Read the model definition and answer for the solid it produces. Units are mm, in the model's axes. A direction names the side the tool comes from. Coordinates: 2 decimals unless noted, no trailing zeros. Write each loop counter-clockwise with the first axis right and the second up, starting at its lowest first coordinate (ties: lowest second). Pieces come first, ordered by that corner, then holes. Notation, with made-up numbers: (-29.75, 55.5) -> (-10.75, 55.5) arc R6 cw to (-10.75, 64.5) -> close; hole circle Ø5 at (-7, -30.5). An arc over 180 degrees is marked (long way). Answer in a Markdown table with one row per item. Add a question column.
Item 1: Straight lines are drawn through the part: line 1 (Y direction, x = 0, z = 182); line 2 (Y direction, x = 12, z = 181.5); line 3 (Y direction, x = 15.75, z = 182.5). For each, find the intervals that lie inside material, in ascending order. Write a range as from..to.
Item 2: Given pin 1 Ø1.5 at (y, z) = (10, 204.5) entering from -X; pin 2 Ø8.5 at (y, z) = (-12.5, 183.5) entering from +X; pin 3 Ø0.5 at (x, z) = (19, 199) entering from -Y; pin 4 Ø2.5 at (x, y) = (-16.5, -11) entering from -Z, each flat-ended and moving along its own axis, determine where each tip first touches the part or whether it passes through.
Item 3: Section A-A on x = 0 is taken. Count the separate pieces of the cut face and the enclosed holes in it, then the cut area to 3 significant figures.
Item 4: Which of the six approach directions +Z, -Z, +X, -X, +Y, -Y give full straight-line access (tool end or side, diameter ignored) to faces 1 (the face through (16, -12, 187.3)), 2 (the face through (22, -7, 182.3)), 3 (the face through (19.069, -3.542, 188.468))?
Item 5: For a pull along Y with two mould halves and no side action, classify faces 4 (the face through (23, 3.7, 196)), 5 (the face through (-23.877, -1.051, 186.742)), 6 (the face through (17, -2, 188)) as +Y half, -Y half, draft (parallel to the pull), parting line (faces both ways), or undercut.
Item 6: Section D-D on z = 201 is taken. Write down the section's boundary in (x, y).
Item 7: Section C-C on z = 205.3 is taken. Write down the section's boundary in (x, y), then the cut area to 3 significant figures.
```python
from build123d import *

# Parameters (mm, degrees)
PAD022_DEPTH    = 10
CHAMFER009_SIZE = 0.5
SKETCH040_R     = 23.9
SKETCH040_R_2   = 22.6
PAD023_DEPTH    = 24
SKETCH041_R     = 23.5
SKETCH041_W     = 20
SKETCH041_H     = 7.75
PAD024_DEPTH    = 24
SKETCH042_R     = 23.9
PAD025_DEPTH    = 4
CHAMFER010_SIZE = 0.5
SKETCH043_R     = 1.5
POCKET013_DEPTH = 15
SKETCH044_R     = 1
POCKET014_DEPTH = 100
SKETCH045_R     = 1.25
POCKET015_DEPTH = 15
SKETCH052_W     = 5
SKETCH052_H     = 18
POCKET019_DEPTH = 41
SKETCH055_W     = 10
SKETCH055_H     = 14
POCKET021_DEPTH = 33


with BuildPart() as part:
    # Sketch039 → Pad022 (new body)
    with BuildSketch(Plane.XY):
        with BuildLine():
            ThreePointArc((-14.5, 18.872997), (-23.8, 0), (-14.5, -18.872997))
            Line((-14.5, -18.872997), (14.5, -18.872997))
            ThreePointArc((14.5, -18.872997), (23.8, 0), (14.5, 18.872997))
            Line((-14.5, 18.872997), (14.5, 18.872997))
        make_face()
        with BuildLine():
            ThreePointArc((-13.831702, 17.872997), (-22.6, 0), (-13.831702, -17.872997))
            Line((13.831702, -17.872997), (-13.831702, -17.872997))
            ThreePointArc((13.831702, -17.872997), (22.6, 0), (13.831702, 17.872997))
            Line((-13.831702, 17.872997), (13.831702, 17.872997))
        make_face(mode=Mode.SUBTRACT)
    extrude(amount=PAD022_DEPTH)

    # Chamfer009
    chamfer009_edges = [part.edges().sort_by_distance(p)[0] for p in [
        (0, -18.872997, 10),
        (0, 18.872997, 10),
    ]]
    chamfer(chamfer009_edges, length=CHAMFER009_SIZE)

    # Sketch040 (on Face4 of Chamfer009) → Pad023 (join)
    with BuildSketch(Plane(origin=(0, 0, 0), x_dir=(1, 0, 0), z_dir=(0, 0, -1))):
        Circle(SKETCH040_R)
        Circle(SKETCH040_R_2, mode=Mode.SUBTRACT)
    extrude(amount=PAD023_DEPTH)

    # Sketch041 (on Face4 of Pad023) → Pad024 (join)
    with BuildSketch(Plane.XY):
        Circle(SKETCH041_R)
        with BuildLine():
            Line((-22.528563, 1.795511), (-18, 0.997003))
            Line((-18, 0.997003), (-18, -0.002997))
            Line((-18, -0.002997), (-20, -0.002997))
            Line((-20, -0.002997), (-20, -2.002997))
            Line((-18, -2.002997), (-20, -2.002997))
            Line((-18, -2.002997), (-18, -3.002997))
            Line((-18, -3.002997), (-22.225594, -4.096705))
            ThreePointArc((-22.225594, -4.096705), (-21.597921, -6.655058), (-20.676821, -9.122997))
            Line((-20.676821, -9.122997), (20.676821, -9.122997))
            ThreePointArc((20.676821, -9.122997), (21.597428, -6.656659), (22.224986, -4.1))
            Line((16, -3), (22.224986, -4.1))
            Line((16, -2), (16, -3))
            Line((18, -2), (16, -2))
            Line((18, 0), (18, -2))
            Line((18, 0), (16, 0))
            Line((16, 0), (16, 1))
            Line((16, 1), (22.528205, 1.8))
            ThreePointArc((22.528205, 1.8), (19.877022, 10.754719), (13.831702, 17.872997))
            Line((13.831702, 17.872997), (-13.831702, 17.872997))
            ThreePointArc((-13.831702, 17.872997), (-19.878094, 10.752739), (-22.528563, 1.795511))
        make_face(mode=Mode.SUBTRACT)
        with Locations((0, -13.997997)):
            Rectangle(SKETCH041_W, SKETCH041_H, mode=Mode.SUBTRACT)
    extrude(amount=-PAD024_DEPTH)

    # Sketch042 (on Face49 of Pad024) → Pad025 (join)
    with BuildSketch(Plane(origin=(0, 0, -24), x_dir=(1, 0, 0), z_dir=(0, 0, -1))):
        Circle(SKETCH042_R)
    extrude(amount=PAD025_DEPTH)

    # Chamfer010
    chamfer010_edges = [part.edges().sort_by_distance(p)[0] for p in [
        (-23.9, 0, -28),
    ]]
    chamfer(chamfer010_edges, length=CHAMFER010_SIZE)

    # Sketch043 (on Face4 of Chamfer010) → Pocket013 (cut)
    with BuildSketch(Plane(origin=(0, 0, -28), x_dir=(1, 0, 0), z_dir=(0, 0, -1))):
        with Locations((-15.75, 11.916375)):
            Circle(SKETCH043_R)
        with Locations((15.75, 11.916375)):
            Circle(SKETCH043_R)
        with Locations((0, -19.75)):
            Circle(SKETCH043_R)
    extrude(amount=-POCKET013_DEPTH, mode=Mode.SUBTRACT)

    # Sketch044 (on Face9 of Pocket013) → Pocket014 (cut)
    with BuildSketch(Plane.XZ.offset(18.872997)):
        with Locations((0, 5)):
            Circle(SKETCH044_R)
    extrude(amount=-POCKET014_DEPTH, mode=Mode.SUBTRACT)

    # Sketch045 (on Face29 of Pocket014) → Pocket015 (cut)
    with BuildSketch(Plane.XY):
        with Locations((12.5, -15)):
            Circle(SKETCH045_R)
        with Locations((-12.5, -15)):
            Circle(SKETCH045_R)
    extrude(amount=-POCKET015_DEPTH, mode=Mode.SUBTRACT)

    # Sketch052 → Pocket019 (cut)
    with BuildSketch(Plane.YZ):
        with Locations((-6.6, -9)):
            Rectangle(SKETCH052_W, SKETCH052_H)
    extrude(amount=POCKET019_DEPTH, mode=Mode.SUBTRACT)

    # Sketch055 → Pocket021 (cut)
    with BuildSketch(Plane.YZ):
        with Locations((8.7, -4.5)):
            Rectangle(SKETCH055_W, SKETCH055_H)
    extrude(amount=POCKET021_DEPTH, mode=Mode.SUBTRACT)


with BuildPart() as part_1:
    # Body017 placement: moved
    add(part.part.moved(Location((0, 0, 200.3))))


solid = part_1.part
```
Results below:
| question | item | result |
|---|---|---|
| 1 | line 1 | y = -23.9..-17.87, -10.12..-9.12, 17.87..18.25, 21.25..23.9 |
| 1 | line 2 | y = -20.67..-9.12, 17.87..20.67 |
| 1 | line 3 | y = -17.98..-13.42, -10.42..-9.12, 16.21..17.98 |
| 2 | pin 1 | stops at x = -21.93 |
| 2 | pin 2 | stops at x = 22.37 |
| 2 | pin 3 | stops at y = -14.82 |
| 2 | pin 4 | stops at z = 172.3 |
| 3 | separate pieces | 3 |
| 3 | enclosed holes | 0 |
| 3 | area | 475 mm2 |
| 4 | face 1 | -Z |
| 4 | face 2 | +X |
| 4 | face 3 | +Z |
| 5 | face 4 | +Y half |
| 5 | face 5 | parting line |
| 5 | face 6 | undercut |
| 6 | outline | (-14.5, -18.87) -> (14.5, -18.87) arc R23.8 ccw to (23.51, 3.7) -> (22.3, 3.7) arc R22.6 cw to (13.83, -17.87) -> (-13.83, -17.87) arc R22.6 cw to (-13.83, 17.87) -> (13.83, 17.87) arc R22.6 cw to (17.97, 13.7) -> (19.46, 13.7) arc R23.8 ccw to (14.5, 18.87) -> (-14.5, 18.87) arc R23.8 ccw to start |
| 7 | outline | (-14.5, -18.87) -> (-1, -18.87) -> (-1, -17.87) -> (-13.83, -17.87) arc R22.6 cw to (-13.83, 17.87) -> (-1, 17.87) -> (-1, 18.87) -> (-14.5, 18.87) arc R23.8 ccw to start; (1, -18.87) -> (14.5, -18.87) arc R23.8 ccw to (14.5, 18.87) -> (1, 18.87) -> (1, 17.87) -> (13.83, 17.87) arc R22.6 cw to (13.83, -17.87) -> (1, -17.87) -> close |
| 7 | area | 154 mm2 |
